Input: part model. Units: mm. Frame: model coordinates. Coordinates: 2 decimals unless noted, no trailing zeros. Order: outer loops, then holes, each group sorted by start corner. A loop starts at its lowest first (then second) coordinate and runs counter-clockwise, first axis right, second up.
from build123d import *

# Parameters (mm, degrees)
SKETCH1_W           = 107.95
SKETCH1_H           = 107.95
BOSS_EXTRUDE1_DEPTH = 3.175
SKETCH2_R           = 2.5527
CUT_EXTRUDE1_DEPTH  = 3.175
SKETCH3_R           = 14.2875
CUT_EXTRUDE2_DEPTH  = 3.175


with BuildPart() as part:
    # Sketch1 → Boss-Extrude1 (new body)
    with BuildSketch(Plane.XY):
        with Locations((53.975, 53.975)):
            Rectangle(SKETCH1_W, SKETCH1_H)
    extrude(amount=BOSS_EXTRUDE1_DEPTH)

    # Sketch2 → Cut-Extrude1 (cut)
    with BuildSketch(Plane(origin=(0, 0, 0), x_dir=(-1, 0, 0), z_dir=(0, 0, -1))):
        with Locations((-6.35, 101.6)):
            Circle(SKETCH2_R)
        with Locations((-101.6, 101.6)):
            Circle(SKETCH2_R)
        with Locations((-101.6, 6.35)):
            Circle(SKETCH2_R)
        with Locations((-6.35, 6.35)):
            Circle(SKETCH2_R)
    extrude(amount=-CUT_EXTRUDE1_DEPTH, mode=Mode.SUBTRACT)

    # Sketch3 → Cut-Extrude2 (cut)
    with BuildSketch(Plane.XY.offset(3.175)):
        with Locations((27.305, 53.975)):
            Circle(SKETCH3_R)
        with Locations((80.645, 53.975)):
            Circle(SKETCH3_R)
    extrude(amount=-CUT_EXTRUDE2_DEPTH, mode=Mode.SUBTRACT)


solid = part.part
Item 1: Pin query (flat end, axial travel): pin 1 Ø6 at (x, y) = (101.6, 101.6) entering from -Z. Return the tip coordinate at first contact, or that it passes through.
Response values:
pin 1: stops at z = 0
Item 2: Ray query, probe 1 along Y at (x, z) = (101.6, 2.1); probe 2 along X at (y, z) = (8, 2.8); probe 3 along X at (y, z) = (55, 0.75). Return the intervals inside material, ascending.
Response values:
probe 1: y = 0 to 3.8, 8.9 to 99.05, 104.15 to 107.95
probe 2: x = 0 to 4.4, 8.3 to 99.65, 103.55 to 107.95
probe 3: x = 0 to 13.05, 41.56 to 66.39, 94.9 to 107.95
Item 3: Cut plane D-D on z = 2.5. Count the separate pieces of the cut face and the enclosed holes in it, then the cut area to 3 significant figures.
Response values:
separate pieces: 1
enclosed holes: 6
area: 10,300 mm2
Item 4: Cut plane A-A on x = 6.35. Return loops of the section in (y, z) (3 decimals).
Response values:
outline: (0, 0) - (3.797, 0) - (3.797, 3.175) - (0, 3.175) - close; (8.903, 0) - (99.047, 0) - (99.047, 3.175) - (8.903, 3.175) - close; (104.153, 0) - (107.95, 0) - (107.95, 3.175) - (104.153, 3.175) - close
Item 5: Draft query along X for faces 1 (the face through (0, 53, 2)), 2 (the face through (53, 55, 3.175)), 3 (the face through (103.63, 4.8, 1.57)). Return one class per face: pulls with the +X half, pulls with the -X half, needs draft (parallel to the pull), parting line crosses it, or undercut.
Response values:
face 1: pulls with the -X half
face 2: needs draft
face 3: undercut
Item 6: Cut plane B-B on y = 49. Return loops of the section in (x, z) (3 decimals), then the cut area to 3 significant figures.
Response values:
outline: (0, 0) - (13.912, 0) - (13.912, 3.175) - (0, 3.175) - close; (40.698, 0) - (67.252, 0) - (67.252, 3.175) - (40.698, 3.175) - close; (94.038, 0) - (107.95, 0) - (107.95, 3.175) - (94.038, 3.175) - close
area: 173 mm2
